```python
from build123d import *

# Parameters (mm, degrees)
FILLET_1_R             = 1
CUT_EXTRUDE_1_DEPTH    = 1
HOLE_WIZARD_M6_1_D     = 5
HOLE_WIZARD_M6_1_DEPTH = 4.1
HOLE_WIZARD_M6_1_TIP   = 1.502151548


with BuildPart() as part:
    # 草图1 → 旋转1 (revolve)
    with BuildSketch(Plane.XY):
        Polygon((0, 0), (0, 6.55), (2.7, 6.55), (2.7, 3.95), (12.7, 3.95), (12.7, 0), align=None)
    revolve(axis=Axis((0, 0, 0), (1, 0, 0)))

    # 圆角1
    fillet_1_edges = [part.edges().sort_by_distance(p)[0] for p in [
        (2.7, -6.55, 0),
        (0, -6.55, 0),
    ]]
    fillet(fillet_1_edges, radius=FILLET_1_R)

    # 草图2 → 切除-拉伸1 (cut)
    with BuildSketch(Plane.ZY):
        Polygon((1.154700538, 2), (-1.154700538, 2), (-2.309401077, 0), (-1.154700538, -2), (1.154700538, -2), (2.309401077, 0), align=None)
    extrude(amount=-CUT_EXTRUDE_1_DEPTH, mode=Mode.SUBTRACT)

    # M6 螺纹孔1
    with Locations(Plane(origin=(12.7, 0, 0), x_dir=(0, 0, -1), z_dir=(1, 0, 0))):
        with Locations((0, 0)):
            Hole(HOLE_WIZARD_M6_1_D / 2, depth=HOLE_WIZARD_M6_1_DEPTH)
            with Locations((0, 0, -(HOLE_WIZARD_M6_1_DEPTH + HOLE_WIZARD_M6_1_TIP / 2))):  # 118° drill point
                Cone(0, HOLE_WIZARD_M6_1_D / 2, HOLE_WIZARD_M6_1_TIP, mode=Mode.SUBTRACT)


solid = part.part
```
Can you work these out from the model? Positions are in its coordinate system, mm. A direction names the side the tool comes from. Coordinates: 2 decimals unless noted, no trailing zeros. Write each loop counter-clockwise with the first axis right and the second up, starting at its lowest first coordinate (ties: lowest second). Pieces come first, ordered by that corner, then holes. Notation, with made-up numbers: M -19.5,62.25 L -14.5,62.25 A12 ccw -14.5,73.25 Z; hole C 38.5,-24 d11. An arc over 180 degrees is marked long. Answer as CSV lines item,"result".
Item 1: Please list where these lines run through material, in increasing order: line 1 along Z through (x, y) = (10, 0); line 2 along Y through (x, z) = (8.75, -1); line 3 along X through (y, z) = (-1, -4.75).
Geometry results:
line 1,"z = -3.95 to -2.5, 2.5 to 3.95"
line 2,"y = -3.82 to -2.29, 2.29 to 3.82"
line 3,"x = 0 to 2.7"
Item 2: Imagine slicing it at A-A on x = 9. List the corners of the cut face in (y, z) for me, plus the area to 3 significant figures.
Geometry results:
outline,"C 0,0 d7.9; hole C 0,0 d5"
area,"29.4 mm2"
Item 3: On a 3-axis mill with a long thin cutter (end or side, diameter ignored), from which of +Z, -Z, +X, -X, +Y, -Y can I reach the whole of each face in a straight line? I mean faces 4 (the cylindrical face through (7.77, -3.135, -2.404)), 5 (the flat face through (0.49, -0.99, -1.74)), 6 (the flat face through (12.7, 0, -3)). Say none if no direction works.
Geometry results:
face 4,"+X"
face 5,"-X"
face 6,"+Z, -Z, +X, +Y, -Y"
Item 4: I'm going to push flat-ended pins straight in: P1, Ø3, axis at x = 6, z = -1.5, coming from the +Y side; P2, Ø4, axis at x = 7, z = -4.5, coming from the +Y side; P3, Ø2, axis at x = 5, y = -4.5, coming from the -Z side. Where does each tip first touch, or does it pass through?
Geometry results:
P1,"stops at y = 3.95"
P2,"stops at y = 3.06"
P3,"stops at z = -1.83"
Item 5: Imagine slicing it at B-B on x = 5.25. List the corners of the cut face in (y, z) for me.
Geometry results:
outline,"C 0,0 d7.9"
Item 6: We'd pull the mould along Z, two halves only. Please class faces 1 (the cylindrical face through (1.355, -0.853, 6.494)), 2 (the conical face through (7.359, -0.424, 0.094)), 3 (the flat face through (0, -2.4, 0.1)): +Z half, -Z half, draft (parallel to the pull), parting line (faces both ways), or undercut.
Geometry results:
face 1,"parting line"
face 2,"undercut"
face 3,"draft"
Item 7: Imagine slicing it at C-C on x = 2.25. List the corners of the cut face in (y, z) for me.
Geometry results:
outline,"C 0,0 d12.77"
